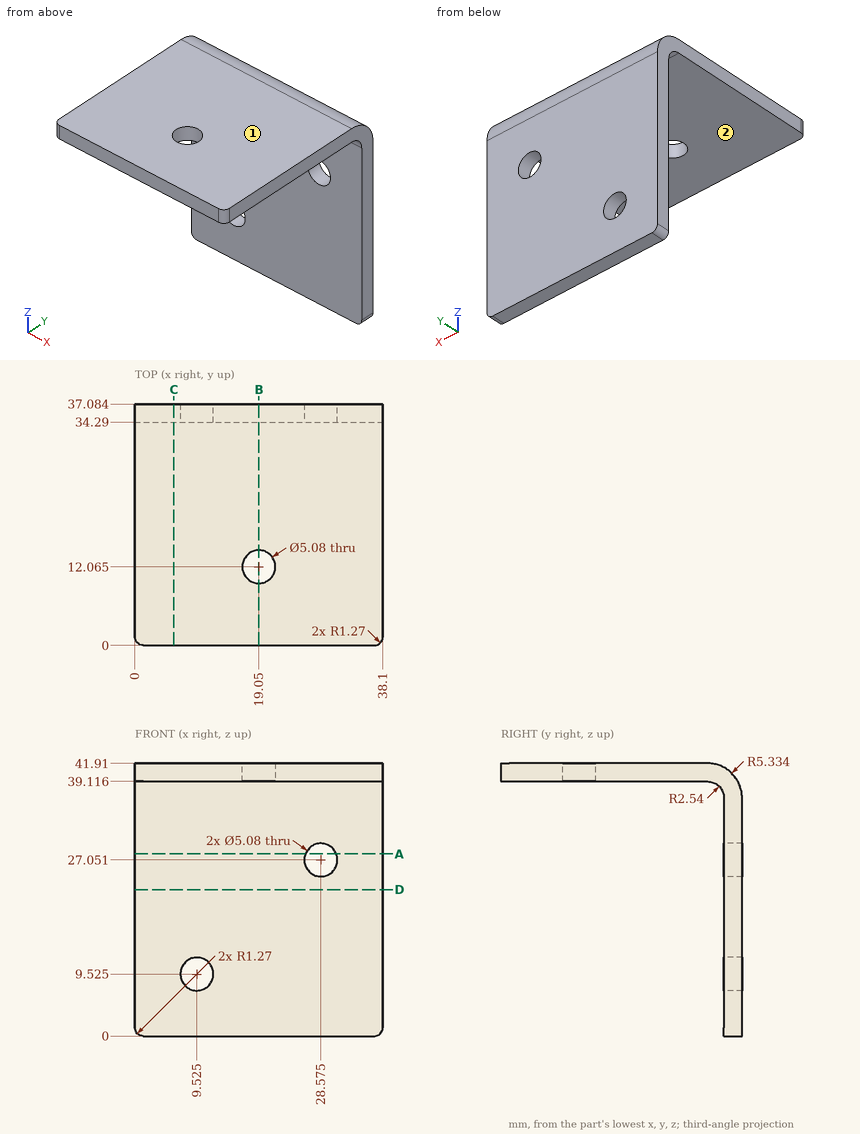
Input: dimensioned drawing with shaded views. Units: mm. Origin: part minimum x, y, z. A direction names the side the tool comes from. Coordinates: 2 decimals unless noted, no trailing zeros. Write each loop counter-clockwise with the first axis right and the second up, starting at its lowest first coordinate (ties: lowest second). Pieces come first, ordered by that corner, then holes. Notation, with made-up numbers: M 77,69 L 94,69 A13 ccw 94,79 Z; hole C 43,75 d7. An arc over 180 degrees is marked long. Answer as a JSON object with one key per item and string values. Group by question number.
(1) Contact query for flat-ended pins moving along their axis: P1, Ø8, axis at y = 15, z = 33.5, coming from the +X side; P2, Ø8, axis at x = 33, z = 23, coming from the -Y side; P3, Ø1, axis at x = 32, y = 21, coming from the -Z side. Output: stop coordinate, or through.
(2) Section D-D on z = 22.5. Output: boundary loops of the cut face in (x, y), plus the area to 3 significant figures.
(3) Section B-B on x = 19.05. Output: boundary loops of the cut face in (y, z) (3 decimals).
(4) Ray query, line 1 along Y through (x, z) = (19.5, 13); line 2 along Z through (x, y) = (13, 8); line 3 along Y through (x, z) = (19.05, 40.85) (3 decimals). Return the intervals inside material, ascending. Write a range as [from, to].
(5) Set-up query: the marked faces 1 and 2. Return all of +Z, -Z, +X, -X, +Y, -Y with unobstructed straight access to the full face (end or side cutting, diameter ignored); none if empty.
(6) Section A-A on z = 28. Output: boundary loops of the cut face in (x, y).
(7) Section C-C on x = 6. Output: boundary loops of the cut face in (y, z), plus the area to 3 significant figures.
Result set:
{
 "1": {"P1": "passes through", "P2": "stops at y = 34.29", "P3": "stops at z = 39.12"},
 "2": {"outline": "M 0,34.29 L 38.1,34.29 L 38.1,37.08 L 0,37.08 Z", "area": "106 mm2"},
 "3": {"outline": "M 0,39.116 L 9.525,39.116 L 9.525,41.91 L 0,41.91 Z; M 14.605,39.116 L 31.75,39.116 A2.54 cw 34.29,36.576 L 34.29,0 L 37.084,0 L 37.084,36.576 A5.334 ccw 31.75,41.91 L 14.605,41.91 Z"},
 "4": {"line 1": "y = [34.29, 37.08]", "line 2": "z = [39.12, 41.91]", "line 3": "y = [0, 9.525], [14.605, 34.941]"},
 "5": {"face 1": "+Z, +X, -X, +Y, -Y", "face 2": "-Z, +X, -X, -Y"},
 "6": {"outline": "M 0,34.29 L 26.22,34.29 L 26.22,37.08 L 0,37.08 Z; M 30.93,34.29 L 38.1,34.29 L 38.1,37.08 L 30.93,37.08 Z"},
 "7": {"outline": "M 0,39.12 L 31.75,39.12 A2.54 cw 34.29,36.58 L 34.29,0 L 37.08,0 L 37.08,36.58 A5.33 ccw 31.75,41.91 L 0,41.91 Z", "area": "208 mm2"}
}
